Design review of the part shown in the three views and the two pictorial views. Dimensions are in mm from the part's minimum x, y and z. Coordinates: 2 decimals unless noted, no trailing zeros. Loops run counter-clockwise (first coordinate to the right, second up) from the corner with the lowest first, then second, coordinate; pieces in that order, holes last. Notation, with made-up numbers: M 37,-25.75 L 54,-25.75 A36 cw 54,11.25 Z; hole C 0.5,63 d3. An arc over 180 degrees is marked long. Put each result on its own line as item: value. Start each with the question number.
(1) Take a section at C-C, the plane z = 191. Give the boundary of the cut face in (x, y) (1 decimal).
(2) Take a section at A-A, the plane x = 152.5. Give the boundary of the cut face in (y, z) (1 decimal), then the cut area to 3 significant figures.
(3) Clearance check with flat-ended pins moving along their axes: pin 1 (8 mm diameter, centred on x = 137, y = 21.5, fed in from -Z); pin 2 (9.5 mm diameter, centred on y = 18.5, z = 552.5, fed in from -X) (3 decimals); pin 3 (18 mm diameter, centred on x = 183.5, y = 13, fed in from -Z); pin 4 (3.5 mm diameter, centred on y = 19, z = 508, fed in from +X) (3 decimals). State where each tip first meets the part, or that it passes through.
(4) For probe 1 along Z at (x, y) = (204.5, 34.5) (1 decimal); probe 2 along X at (y, z) = (14.5, 700) (1 decimal), list the stretches that pass through material, from the lowest coordinate up. Write a range as [from, to].
(5) Take a section at B-B, the plane y = 6. Give the boundary of the cut face in (x, z) (1 decimal), then the cut area to 3 significant figures.
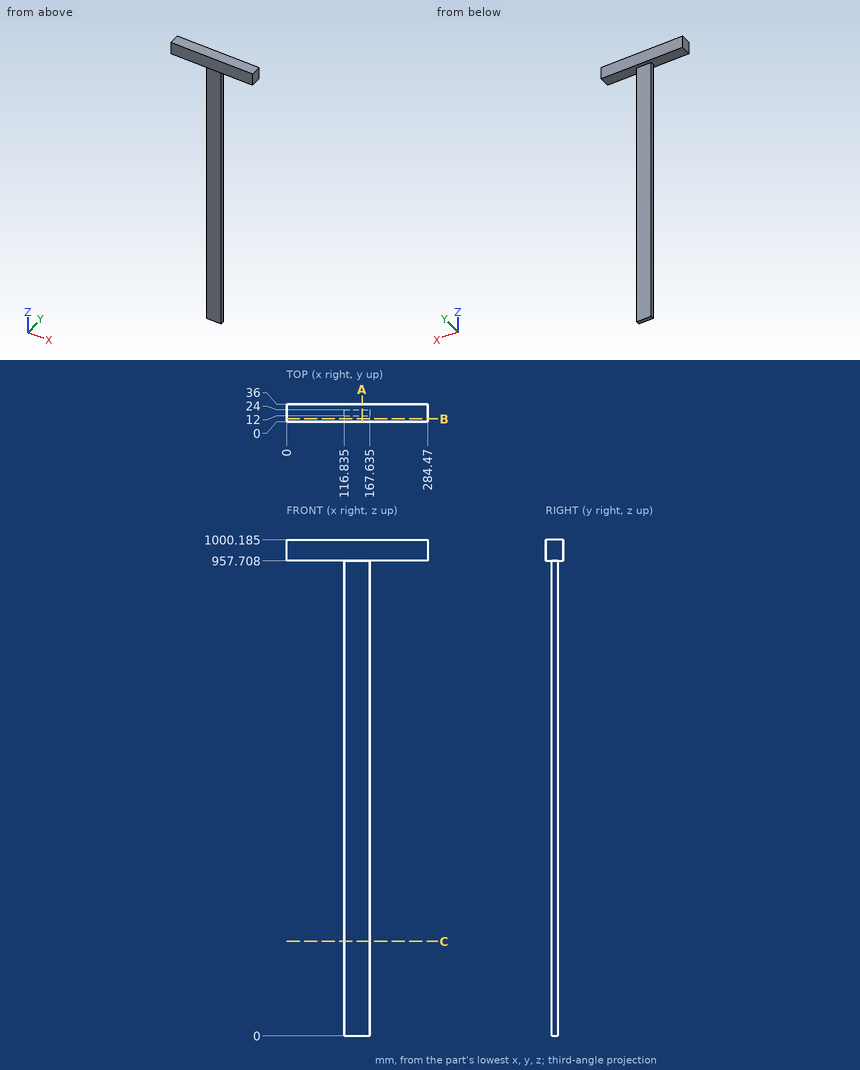
Computed values:
1. outline: M 116.8,12 L 167.6,12 L 167.6,24 L 116.8,24 Z
2. outline: M 0,957.7 L 12,957.7 L 12,0 L 24,0 L 24,957.7 L 36,957.7 L 36,1000.2 L 0,1000.2 Z
2. area: 13,000 mm^2
3. pin 1: stops at z = 0
3. pin 2: stops at x = 116.835
3. pin 3: stops at z = 957.71
3. pin 4: stops at x = 167.635
4. probe 1: z = [957.7, 1000.2]
4. probe 2: x = [116.8, 167.6]
5. outline: M 0,957.7 L 284.5,957.7 L 284.5,1000.2 L 0,1000.2 Z
5. area: 12,100 mm^2
